CAD build for the part. Positions are in the model's coordinates, mm. Face numbers are marked on the shaded views. Coordinates: 2 decimals unless noted, no trailing zeros. Write each loop counter-clockwise with the first axis right and the second up, starting at its lowest first coordinate (ties: lowest second). Pieces come first, ordered by that corner, then holes. Notation, with made-up numbers: M 16,-9 L 41,-9 A21 ccw 41,22 Z; hole C 14,24 d3. An arc over 180 degrees is marked long. Put each result on its own line as item: value. Start each with the question number.
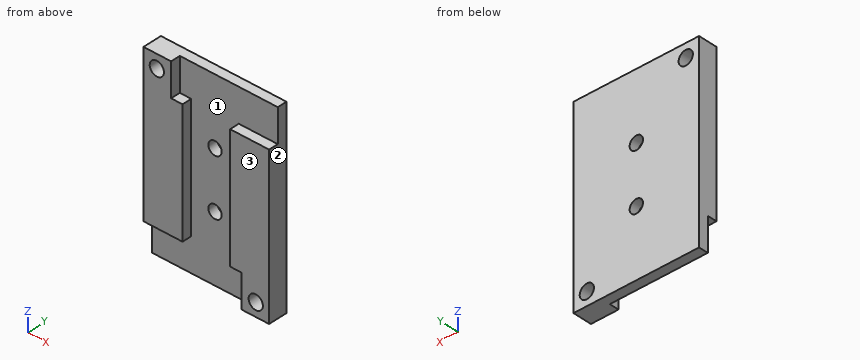
```python
from build123d import *

# Parameters (mm, degrees)
SKETCH_1_W          = 13.2
SKETCH_1_H          = 20
EXTRUDE_1_DEPTH     = 2
SKETCH_1_3_R        = 0.75
CUT_EXTRUDE_2_DEPTH = 13.147427711
CUT_EXTRUDE_START   = -2
CUT_EXTRUDE_1_DEPTH = 1
SKETCH_2_4_R        = 0.7
CUT_EXTRUDE_3_DEPTH = 13.147427711


with BuildPart() as part:
    # 草图1 → 凸台-拉伸1 (new body)
    with BuildSketch(Plane(origin=(0, 0, 0), x_dir=(1, 0, 0), z_dir=(0, 1, 0))):
        Rectangle(SKETCH_1_W, SKETCH_1_H)
    extrude(amount=EXTRUDE_1_DEPTH)

    # 草图1<3> → 切除-拉伸2 (cut, through all)
    with BuildSketch(Plane(origin=(0, 0, 0), x_dir=(1, 0, 0), z_dir=(0, 1, 0))):
        with Locations(Location((-5.2, -8.6, 0), (0, 0, 270))):
            Circle(SKETCH_1_3_R)
        with Locations(Location((5.2, 8.6, 0), (0, 0, 270))):
            Circle(SKETCH_1_3_R)
    extrude(amount=CUT_EXTRUDE_2_DEPTH, mode=Mode.SUBTRACT)

    # 草图2 → 切除-拉伸1 (cut)
    with BuildSketch(Plane(origin=(0, 2, 0), x_dir=(1, 0, 0), z_dir=(0, 1, 0)).offset(CUT_EXTRUDE_START)):
        Polygon((3.7, 10), (-6.6, 10), (-6.6, 6.5), (-2.5, 6.5), (-2.5, -6.5), (-3.7, -6.5), (-3.7, -10), (6.6, -10), (6.6, -6.5), (2.5, -6.5), (2.5, 6.5), (3.7, 6.5), align=None)
    extrude(amount=CUT_EXTRUDE_1_DEPTH, mode=Mode.SUBTRACT)

    # 草图2<4> → 切除-拉伸3 (cut, through all)
    with BuildSketch(Plane(origin=(0, 2, 0), x_dir=(1, 0, 0), z_dir=(0, 1, 0))):
        with Locations(Location((0, 3, 0), (0, 0, 270))):
            Circle(SKETCH_2_4_R)
        with Locations(Location((0, -3, 0), (0, 0, 270))):
            Circle(SKETCH_2_4_R)
    extrude(amount=-CUT_EXTRUDE_3_DEPTH, mode=Mode.SUBTRACT)


solid = part.part
```
(1) Slice it at B-B, the plane x = 5.2. Write the cut outline in (y, z), then the cut area to 3 significant figures.
(2) Two-plate mould, pull along X, no slides. Class the marked faces 1, 2 and 3: +X half, -X half, draft (parallel to the pull), parting line (faces both ways), or undercut.
(3) Slice it at A-A, the plane z = 8.6. Write the cut outline in (x, y), then the cut area to 3 significant figures.
(4) Drill centre lines: line 1 (Z direction, x = 5.2, y = 1.3); line 2 (X direction, y = 0.55, z = 0); line 3 (Z direction, x = -5.25, y = 0.55). Where is each one in solid material? Low to high. Write a range as [from, to].
(5) Slice it at C-C, the plane y = 1.6. Write the cut outline in (x, z), then the cut area to 3 significant figures.
(6) Slice it at D-D, the plane x = 0. Write the cut outline in (y, z).
(7) Drop flat-ended pins along their axis: pin 1 (0.8 mm diameter, centred on x = 5, y = 0.5, fed in from +Z); pin 2 (0.5 mm diameter, centred on y = 0.5, z = -8, fed in from -X); pin 3 (0.8 mm diameter, centred on x = -4, y = 0.5, fed in from -Z). Give the stop position or say it passes through.
Result set:
1. outline: M 0,-10 L 2,-10 L 2,-9.35 L 0,-9.35 Z; M 0,-7.85 L 2,-7.85 L 2,10 L 1,10 L 1,6.5 L 0,6.5 Z
1. area: 33.5 mm^2
2. face 1: undercut
2. face 2: +X half
2. face 3: draft
3. outline: M -6.6,0 L -5.95,0 L -5.95,2 L -6.6,2 Z; M -4.45,0 L -3.7,0 L -3.7,1 L 6.6,1 L 6.6,2 L -4.45,2 Z
3. area: 13.1 mm^2
4. line 1: z = [-10, -9.35], [-7.85, 10]
4. line 2: x = [-6.6, -2.5], [2.5, 6.6]
4. line 3: z = [-6.5, 7.85], [9.35, 10]
5. outline: M -6.6,-10 L 6.6,-10 L 6.6,10 L -6.6,10 Z; hole C -5.2,8.6 d1.5; hole C 0,-3 d1.4; hole C 0,3 d1.4; hole C 5.2,-8.6 d1.5
5. area: 257 mm^2
6. outline: M 1,-10 L 2,-10 L 2,-3.7 L 1,-3.7 Z; M 1,-2.3 L 2,-2.3 L 2,2.3 L 1,2.3 Z; M 1,3.7 L 2,3.7 L 2,10 L 1,10 Z
7. pin 1: stops at z = 6.5
7. pin 2: stops at x = 3.7
7. pin 3: stops at z = -6.5
